The listing builds one solid part. Answer for the finished solid, in the listing's coordinates (mm). A direction names the side the tool comes from. Coordinates: 2 decimals unless noted, no trailing zeros. Order: outer loops, then holes, each group sorted by start corner. A loop starts at its lowest first (then second) coordinate and runs counter-clockwise, first axis right, second up.
Autodesk Inventor part; units mm, degrees
ref_plane "YZ Plane" through (0, 0, 0) normal (1, 0, 0) x (0, 1, 0)
ref_plane "XZ Plane" through (0, 0, 0) normal (0, 1, 0) x (-1, 0, 0)
ref_plane "XY Plane" through (0, 0, 0) normal (0, 0, 1) x (1, 0, 0)
sketch "Эскиз1" plane through (0, 0, 0) normal (0, 0, 1) x (1, 0, 0)
  circle A0 centre (0, 0) radius 60 construction
  line L0 (-80, -70) -> (-80, -50)
  line L1 (-80, -50) -> (-30, 8)
  line L2 (-30, 8) -> (72, 8)
  line L3 (72, 8) -> (90, -50)
  line L4 (90, -50) -> (90, -70)
  line L5 (90, -70) -> (-80, -70)
  line L6 (0, -110.4) -> (0, 88.4) construction
  line L7 (-115.4, 0) -> (132.4, 0) construction
  line L8 (-80, -50) -> (90, -50) construction
  circle A1 centre (67, -35) radius 12.5 construction
  circle A2 centre (0, 0) radius 5.1
  circle A3 centre (66, 0) radius 4.1
  circle A4 centre (67, -35) radius 4
  circle A5 centre (67, -35) radius 8.5 construction
  line L9 (67, -49.1463) -> (67, -22.5) construction
  circle A6 centre (67, -43.5) radius 1.6
  circle A7 centre (67, -26.5) radius 1.6
  line L10 (-24.5014, -4) -> (-68, -54.4584)
  line L11 (-68, -54.4584) -> (-68, -58)
  line L12 (-68, -58) -> (78, -58)
  line L13 (78, -58) -> (78, -51.8193)
  line L14 (78, -51.8193) -> (63.1595, -4)
  line L15 (63.1595, -4) -> (-24.5014, -4)
  arc A8 (-3.5925, -14.5634) -> (14.4568, -4) centre (0, 0) ccw
  arc A9 (-14.4568, -4) -> (-3.5925, -14.5634) centre (0, 0) ccw
  arc A10 (14.4568, -4) -> (-14.4568, -4) centre (0, 0) ccw construction
  line L16 (-9, -58) -> (-9, -12)
  line L17 (9, -58) -> (9, -12)
  arc A11 (65.0062, -9.9505) -> (56.8348, -4) centre (66, 0) ccw construction
  line L18 (68.4354, -21) -> (58.4354, -21)
  line L19 (58.4354, -21) -> (47.8258, -58)
  arc A12 (56.8348, -4) -> (65.0062, -9.9505) centre (66, 0) ccw
  line L20 (-80, -70) -> (-80, -82)
  line L21 (-80, -82) -> (-60, -82)
  line L22 (-60, -82) -> (-60, -70)
  line L23 (90, -70) -> (90, -82)
  line L24 (90, -82) -> (70, -82)
  line L25 (70, -82) -> (70, -70)
  circle A13 centre (-71, -66) radius 4
  circle A14 centre (81, -66) radius 4
  line L26 (-80, -66) -> (90, -66) construction
  line L27 (-5.1, 0) -> (-5.1, 8)
  line L28 (5.1, 0) -> (5.1, 8)
  circle A15 centre (37.4657, -40.2656) radius 6
  circle A16 centre (37.4657, -40.2656) radius 12
  circle A17 centre (67, -35) radius 30 construction
  circle A18 centre (0, 0) radius 55 construction
  line L29 (9, -40.2656) -> (74.4144, -40.2656) construction
  line L30 (9, -47.2656) -> (50.9039, -47.2656)
  line L31 (9, -33.2656) -> (54.9183, -33.2656)
  line L32 (69.7458, -32.0913) -> (70, -32.0913)
  circle A19 centre (0, 0) radius 10.05 construction
  circle A20 centre (-10.05, 0) radius 1.5
  circle A21 centre (10.05, 0) radius 1.5
  circle A22 centre (0, -10.05) radius 1.5
  circle A23 centre (-39, -66) radius 12
  circle A24 centre (-39, -66) radius 6
  point P0 (56.8348, -4)
  point P1 (65.0062, -9.9505)
  point P2 (59.5152, -7.6123)
  point P3 (27.7189, -33.2656)
  point P4 (27.7189, -47.2656)
  point P5 (47.2125, -47.2656)
  point P6 (47.2125, -33.2656)
  point P7 (3.1639, -4)
  point P8 (-3.1639, -4)
  point P9 (-27.6863, -70)
  point P10 (-50.3137, -70)
  point P11 (-30.0557, -58)
  point P12 (-47.9443, -58)
  dimension "d0" = 120
  dimension "d1" = 25
  dimension "d14" = 8
  dimension "d44" = 60
  dimension "d45" = 110
  dimension "d2" = 10.2
  dimension "d3" = 8
  dimension "d5" = 20
  dimension "d6" = 70
  dimension "d8" = 30
  dimension "d9" = 72
  dimension "d10" = 8.2
  dimension "d11" = 66
  dimension "d12" = 80
  dimension "d13" = 90
  dimension "d15" = 35
  dimension "d17" = 17
  dimension "d19" = 3.2
  dimension "d20" = 67
  dimension "d25" = 12
  dimension "d26" = 30
  dimension "d27" = 9
  dimension "d28" = 9
  dimension "d29" = 20
  dimension "d31" = 21
  dimension "d32" = 106
  dimension "d33" = 10
  dimension "d35" = 20
  dimension "d36" = 12
  dimension "d37" = 8
  dimension "d38" = 8
  dimension "d39" = 16
  dimension "d40" = 9
  dimension "d41" = 9
  dimension "d42" = 12
  dimension "d43" = 24
  dimension "d47" = 7
  dimension "d48" = 7
  dimension "d52" = 3
  dimension "d53" = 3
  dimension "d54" = 3
  dimension "d55" = 20.1
  dimension "d56" = 24
  dimension "d57" = 12
  dimension "d58" = 32
extrude "Выдавливание1" add sketch "Эскиз1" along normal blind 6 contours L0 L1 L2 L27 A2 L15 L10 L11 L12 A23 L5 | L5 L22 L21 L20 | A23 L12 L5 A24 | L5 A24 A23 | L2 L3 L4 L5 A23 L12 L13 L14 L15 A2 L28 | A23 L12 | A2 L15 A8 A9 | L5 L23 L24 L25 | L16 A9 A8 L17 L12 | L15 L14 A12
fillet "Сопряжение1" radius 4 24 edges at (9, -12, 3) (-24.5014, -4, 3) (-9, -58, 3) (-68, -54.4584, 3) (-68, -58, 3) (9, -58, 3) (56.8348, -4, 3) (65.0062, -9.9505, 3) (-80, -82, 3) (-60, -82, 3) (-60, -70, 3) (70, -70, 3) (70, -82, 3) (90, -82, 3) (5.1, 8, 3) (-5.1, 8, 3) (78, -58, 3) (-14.4568, -4, 3) (-9, -12, 3) (14.4568, -4, 3) (-47.9443, -58, 3) (-30.0557, -58, 3) (-50.3137, -70, 3) (-27.6863, -70, 3)
fillet "Сопряжение1" radius 20 3 edges at (-80, -50, 3) (-30, 8, 3) (90, -50, 3)
fillet "Сопряжение1" radius 8 2 edges at (72, 8, 3) (78, -51.8193, 3)
equation "\"d28\" = d27"
properties part number "Опора катушки (врунтренняя)"
(1) For faces 1 (the face through (-6.241, 6.797, 3.042)), 2 (the face through (-70, -82, 3)), 3 (the face through (-54, -70, 3)), 4 (the face through (-78.859, -80.797, 3.042)), 5 (the face through (-56, -58, 3)), determine the directions among +Z, -Z, +X, -X, +Y, -Y from which every point of the face is accessible in a straight line to the end or side of a thin tool.
(2) Find section D-D (z = 1). Give the number of separate pieces and of enclosed holes in the cut face, and give its area (3 significant figures).
(3) Find section B-B (x = 48.5). Write down the section's boundary in (y, z), and give its area (3 significant figures).
(4) Consider line 1 (X direction, y = -39, z = 4); line 2 (X direction, y = -66, z = 1.8); line 3 (Y direction, x = 31.5, z = 1.75). Determine where each line is inside the solid, lowest interval first.
(5) Find section C-C (x = -39). Write down the section's boundary in (y, z), and give its area (3 significant figures).
(6) The mould has two halves that part along Y. Classify faces 6 (the face through (-45.25, -28.07, 2.96)), 7 (the face through (-80, -68, 3)), 8 (the face through (-78.713, -50.372, 3.042)): released by +Y, released by -Y, zero draft, split by the parting line, or undercut.
(7) Find section A-A (y = -66). Write down the section's boundary in (x, z).
(8) Each of these flat-tipped pins is pushed along its axis until it touches: pin 1 Ø3 at (y, z) = (-2, 3) entering from -X; pin 2 Ø1.6 at (x, z) = (-54, 3.5) entering from -Y; pin 3 Ø1.2 at (y, z) = (2, 3) entering from -X. Where does it stop, or does it pass through?
Findings below:
1. face 1: +Z, -Z, +Y
1. face 2: +Z, -Z, +X, -X, -Y
1. face 3: +Z, -Z, -Y
1. face 4: +Z, -Z, -X, -Y
1. face 5: +Z, -Z
2. separate pieces: 1
2. enclosed holes: 9
2. area: 6,150 mm2
3. outline: (-70, 0) - (-58, 0) - (-58, 6) - (-70, 6) - close; (-4, 0) - (8, 0) - (8, 6) - (-4, 6) - close
3. area: 144 mm2
4. line 1: x = -70.52 to -54.67, -9 to 9, 74.02 to 86.59
4. line 2: x = -80 to -75, -67 to -45, -33 to 77, 85 to 90
4. line 3: y = -70 to -58, -4 to 8
5. outline: (-78, 0) - (-72, 0) - (-72, 6) - (-78, 6) - close; (-60, 0) - (-54, 0) - (-54, 6) - (-60, 6) - close; (-20.82, 0) - (-2.44, 0) - (-2.44, 6) - (-20.82, 6) - close
5. area: 182 mm2
6. face 6: undercut
6. face 7: zero draft
6. face 8: released by +Y
7. outline: (-80, 0) - (-75, 0) - (-75, 6) - (-80, 6) - close; (-67, 0) - (-45, 0) - (-45, 6) - (-67, 6) - close; (-33, 0) - (77, 0) - (77, 6) - (-33, 6) - close; (85, 0) - (90, 0) - (90, 6) - (85, 6) - close
8. pin 1: stops at x = -39.91
8. pin 2: stops at y = -70
8. pin 3: stops at x = -35.68
